Can you work these out from the model? Positions are in its coordinate system, mm. Give positions to 0.01 mm unless a question says otherwise; leave off trailing zeros. Loops run counter-clockwise (first coordinate to the right, second up) from the corner with the lowest first, then second, coordinate; pieces in that order, holes last. Notation, with made-up numbers: (66, 53.25) - (73, 53.25) arc R32 cw to (73, 85.25) - close; hole circle Ø6 at (34.25, 86). An arc over 180 degrees is marked (long way). Answer as a JSON object with one key per item and string values. Group by question number.
Item 1: Suppose I cut it at C-C on z = 2.75. Count the separate pieces of the cut face and the enclosed holes in it, and give its area (3 significant figures).
Item 2: Suppose I cut it at B-B on y = 0. Write out the boundary of the cut face in (x, z) (3 decimals), and give its area (3 significant figures).
Item 3: Suppose I cut it at D-D on y = 118. Write out the boundary of the cut face in (x, z).
Item 4: Please list where these lines run through material, in increasing order: L1, parallel to Y at x = -1, z = 2.15; L2, parallel to X at y = 169, z = 1.85; L3, parallel to X at y = 82, z = 1.4.
Item 5: Will these pins go through, and if not, where does the flat tip stop? pin 1 (4 mm diameter, centred on x = 19, y = -8, fed in from +Z); pin 2 (1.5 mm diameter, centred on y = 39, z = 2, fed in from +X); pin 3 (2.5 mm diameter, centred on y = 123, z = 2, fed in from +X); pin 4 (2 mm diameter, centred on y = 85.5, z = 2, fed in from +X).
Item 6: Suppose I cut it at A-A on x = -31. Write out the boundary of the cut face in (y, z) (3 decimals).
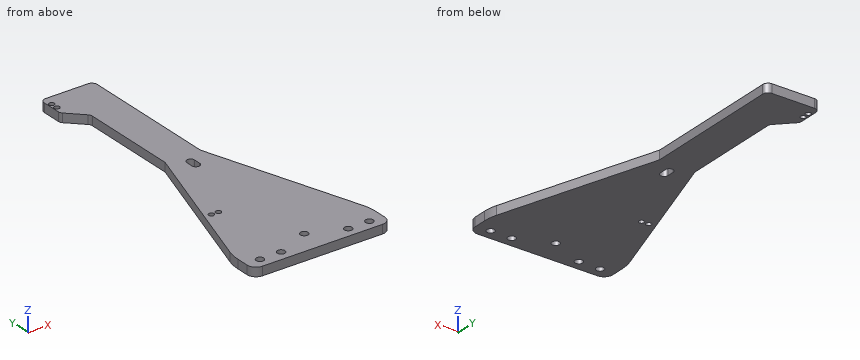
from build123d import *

# Parameters (mm, degrees)
SKETCH_R   = 2.175
SKETCH_R_2 = 1.5
PAD_DEPTH  = 5
FILLET_R   = 3


with BuildPart() as part:
    # Sketch → Pad (new body)
    with BuildSketch(Plane.XY):
        with BuildLine():
            Line((-34, -14), (34, -14))
            ThreePointArc((34, -14), (37.535534, -12.535534), (39, -9))
            Line((39, -9), (39, -1.887209))
            ThreePointArc((39, -1.887209), (38.703164, 1.953845), (37.819704, 5.703686))
            Line((10, 93), (37.819704, 5.703686))
            Line((10, 93), (10, 175))
            Line((-10, 175), (10, 175))
            Line((-10, 175), (-20, 175))
            Line((-20, 175), (-20, 160))
            Line((-20, 160), (-10, 150))
            Line((-10, 93), (-10, 150))
            Line((-37.819704, 5.703686), (-10, 93))
            ThreePointArc((-37.819704, 5.703686), (-38.703164, 1.953845), (-39, -1.887209))
            Line((-39, -9), (-39, -1.887209))
            ThreePointArc((-39, -9), (-37.535534, -12.535534), (-34, -14))
        make_face()
        Circle(SKETCH_R, mode=Mode.SUBTRACT)
        with Locations((19, -8)):
            Circle(SKETCH_R, mode=Mode.SUBTRACT)
        with Locations((31, -8)):
            Circle(SKETCH_R, mode=Mode.SUBTRACT)
        with Locations((-19, -8)):
            Circle(SKETCH_R, mode=Mode.SUBTRACT)
        with Locations((-31, -8)):
            Circle(SKETCH_R, mode=Mode.SUBTRACT)
        with Locations((-19, 40)):
            Circle(SKETCH_R_2, mode=Mode.SUBTRACT)
        with Locations((-23, 40)):
            Circle(SKETCH_R_2, mode=Mode.SUBTRACT)
        with Locations((-18, 165)):
            Circle(SKETCH_R_2, mode=Mode.SUBTRACT)
        with Locations((-18, 169)):
            Circle(SKETCH_R_2, mode=Mode.SUBTRACT)
        with BuildLine():
            ThreePointArc((2.175, 87), (0, 89.175), (-2.175, 87))
            Line((-2.175, 87), (-2.175, 83))
            ThreePointArc((-2.175, 83), (1e-06, 80.825), (2.175, 83.000002))
            Line((2.175, 83.000002), (2.175, 87))
        make_face(mode=Mode.SUBTRACT)
    extrude(amount=PAD_DEPTH)

    # Fillet
    fillet_edges = [part.edges().sort_by_distance(p)[0] for p in [
        (-20, 175, 2.5),
        (10, 175, 2.5),
        (-10, 150, 2.5),
        (-20, 160, 2.5),
    ]]
    fillet(fillet_edges, radius=FILLET_R)


solid = part.part
Worked out:
{
 "1": {"separate pieces": "1", "enclosed holes": "10", "area": "7,400 mm2"},
 "2": {"outline": "(-38.929, 0) - (-2.175, 0) - (-2.175, 5) - (-38.929, 5) - close; (2.175, 0) - (38.929, 0) - (38.929, 5) - (2.175, 5) - close", "area": "368 mm2"},
 "3": {"outline": "(-10, 0) - (10, 0) - (10, 5) - (-10, 5) - close"},
 "4": {"L1": "y = -14 to -1.93, 1.93 to 81.07, 88.93 to 175", "L2": "x = -20 to -19.5, -16.5 to 10", "L3": "x = -13.51 to -1.93, 1.93 to 13.51"},
 "5": {"pin 1": "passes through", "pin 2": "stops at x = 27.45", "pin 3": "stops at x = 10", "pin 4": "stops at x = 12.71"},
 "6": {"outline": "(-14, 0) - (-10.175, 0) - (-10.175, 5) - (-14, 5) - close; (-5.825, 0) - (27.103, 0) - (27.103, 5) - (-5.825, 5) - close"}
}
